Input: part model. Units: mm. Frame: model coordinates. Face numbers are marked on the shaded views. A direction names the side the tool comes from. Coordinates: 2 decimals unless noted, no trailing zeros. Loops run counter-clockwise (first coordinate to the right, second up) from the corner with the lowest first, then second, coordinate; pieces in that order, holes last. Notation, with made-up numbers: M 5.5,10 L 37.5,10 A17 ccw 37.5,41 Z; hole C 38.5,23.5 d10. An arc over 180 degrees is marked long. Use a Markdown table: item, result. Add a question column.
1. Section A-A on z = 0. Output: boundary loops of the cut face in (x, y), then the cut area to 3 significant figures.
2. Set-up query: the marked faces 4 and 5. Return all of +Z, -Z, +X, -X, +Y, -Y with unobstructed straight access to the full face (end or side cutting, diameter ignored); none if empty.
3. Line query: L1, parallel to X at y = 2.3, z = 0; L2, parallel to Z at x = 6, y = 2.45; L3, parallel to Y at x = 6.5, z = -6. Output: solid intervals per line, ascending. Write a range as [from, to].
4. Section C-C on y = 2.5. Output: boundary loops of the cut face in (x, z).
5. Draft query along X for the marked faces 1, 2 and 3. Return one class per face: +X half, -X half, draft (parallel to the pull), parting line (faces both ways), or undercut.
6. Section D-D on z = 3.5. Output: boundary loops of the cut face in (x, y).
7. Pin query (flat end, axial travel): pin 1 (12 mm diameter, centred on x = 5.5, z = 7, fed in from -Y); pin 2 (1 mm diameter, centred on x = -2.5, z = -0.5, fed in from +Y); pin 3 (4 mm diameter, centred on y = 16, z = -8, fed in from +X). Return the tip coordinate at first contact, or that it passes through.
8. Section B-B on x = -1. Output: boundary loops of the cut face in (y, z), then the cut area to 3 significant figures.
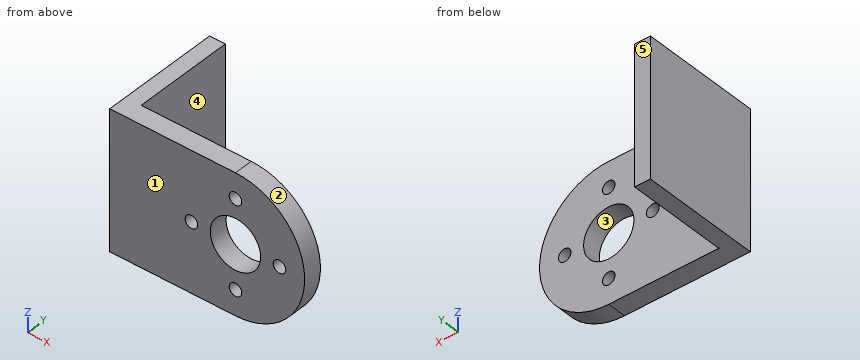
```python
from build123d import *

# Parameters (mm, degrees)
SKETCH1_R           = 1
SKETCH1_R_2         = 4
BOSS_EXTRUDE1_DEPTH = 3
SKETCH2_W           = 2.5
SKETCH2_H           = 22
BOSS_EXTRUDE2_DEPTH = 16


with BuildPart() as part:
    # Sketch1 → Boss-Extrude1 (new body)
    with BuildSketch(Plane(origin=(0, 0, 0), x_dir=(1, 0, 0), z_dir=(0, 1, 0))):
        with BuildLine():
            Line((-14, -11), (-14, 11))
            Line((-14, 11), (6, 11))
            ThreePointArc((6, 11), (17, 0), (6, -11))
            Line((6, -11), (-14, -11))
        make_face()
        with Locations((6, -7)):
            Circle(SKETCH1_R, mode=Mode.SUBTRACT)
        with Locations((-1, 0)):
            Circle(SKETCH1_R, mode=Mode.SUBTRACT)
        with Locations((6, 0)):
            Circle(SKETCH1_R_2, mode=Mode.SUBTRACT)
        with Locations((13, 0)):
            Circle(SKETCH1_R, mode=Mode.SUBTRACT)
        with Locations((6, 7)):
            Circle(SKETCH1_R, mode=Mode.SUBTRACT)
    extrude(amount=BOSS_EXTRUDE1_DEPTH)

    # Sketch2 → Boss-Extrude2 (add)
    with BuildSketch(Plane(origin=(0, 3, 0), x_dir=(1, 0, 0), z_dir=(0, 1, 0))):
        with Locations((-12.75, 0)):
            Rectangle(SKETCH2_W, SKETCH2_H)
    extrude(amount=BOSS_EXTRUDE2_DEPTH)


solid = part.part
```
Answers below:
| question | item | result |
|---|---|---|
| 1 | outline | M -14,0 L -2,0 L -2,3 L -11.5,3 L -11.5,19 L -14,19 Z; M 0,0 L 2,0 L 2,3 L 0,3 Z; M 10,0 L 12,0 L 12,3 L 10,3 Z; M 14,0 L 17,0 L 17,3 L 14,3 Z |
| 1 | area | 97.0 mm² |
| 2 | face 4 | +Z, -Z, +X, +Y |
| 2 | face 5 | +Z, -Z, +X, -X, +Y |
| 3 | L1 | x = [-14, -2], [0, 2], [10, 12], [14, 17] |
| 3 | L2 | z = [-11, -8], [-6, -4], [4, 6], [8, 11] |
| 3 | L3 | y = [0, 3] |
| 4 | outline | M -14,-11 L 6,-11 A11 ccw 6,11 L -14,11 Z; hole C -1,0 d2; hole C 6,0 d8; hole C 6,-7 d2; hole C 6,7 d2; hole C 13,0 d2 |
| 5 | face 1 | draft |
| 5 | face 2 | +X half |
| 5 | face 3 | undercut |
| 6 | outline | M -14,0 L 4.06,0 L 4.06,3 L -11.5,3 L -11.5,19 L -14,19 Z; M 7.94,0 L 16.43,0 L 16.43,3 L 7.94,3 Z |
| 7 | pin 1 | stops at y = 0 |
| 7 | pin 2 | stops at y = 3 |
| 7 | pin 3 | stops at x = -11.5 |
| 8 | outline | M 0,-11 L 3,-11 L 3,-1 L 0,-1 Z; M 0,1 L 3,1 L 3,11 L 0,11 Z |
| 8 | area | 60.0 mm² |
